Autodesk Inventor part; units mm, degrees
ref_plane "YZ Plane" through (0, 0, 0) normal (1, 0, 0) x (0, 1, 0)
ref_plane "XZ Plane" through (0, 0, 0) normal (0, 1, 0) x (-1, 0, 0)
ref_plane "XY Plane" through (0, 0, 0) normal (0, 0, 1) x (1, 0, 0)
sketch "Sketch1" plane through (0, 0, 0) normal (0, 1, 0) x (-1, 0, 0)
  line L0 (0, 0) -> (130, 0)
  line L1 (130, 0) -> (130, -100)
  line L2 (130, -100) -> (0, -100)
  line L3 (0, -100) -> (0, 0)
  dimension "d0" = 130
  dimension "d1" = 100
extrude "Extrusion1" add sketch "Sketch1" along normal blind 8
sketch "Sketch3" plane through (0, 8, 0) normal (0, 1, 0) x (1, 0, 0)
  line L0 (-120, 5) -> (-110, 5)
  line L1 (-110, 5) -> (-110, 15)
  line L2 (-110, 15) -> (-120, 15)
  line L3 (-120, 15) -> (-120, 5)
  line L4 (-130, 100) -> (-130, 0)
  line L5 (-130, 0) -> (0, 0)
  line L6 (-105, 0) -> (-105, 100)
  line L7 (0, 100) -> (-130, 100)
  line L8 (-130, 20) -> (-105, 20)
  line L9 (-120, 35) -> (-110, 35)
  line L10 (-110, 35) -> (-110, 25)
  line L11 (-110, 25) -> (-120, 25)
  line L12 (-120, 25) -> (-120, 35)
  line L13 (-130, 40) -> (-105, 40)
  line L14 (-120, 75) -> (-110, 75)
  line L15 (-110, 75) -> (-110, 65)
  line L16 (-110, 65) -> (-120, 65)
  line L17 (-120, 65) -> (-120, 75)
  line L18 (-120, 45) -> (-110, 45)
  line L19 (-110, 45) -> (-110, 55)
  line L20 (-110, 55) -> (-120, 55)
  line L21 (-120, 55) -> (-120, 45)
  line L22 (-130, 80) -> (-105, 80)
  line L23 (-120, 155) -> (-110, 155)
  line L24 (-110, 155) -> (-110, 145)
  line L25 (-110, 145) -> (-120, 145)
  line L26 (-120, 145) -> (-120, 155)
  line L27 (-130, 100) -> (0, 100)
  line L28 (-120, 125) -> (-110, 125)
  line L29 (-110, 125) -> (-110, 135)
  line L30 (-110, 135) -> (-120, 135)
  line L31 (-120, 135) -> (-120, 125)
  line L32 (-110, 95) -> (-120, 95)
  line L33 (-120, 95) -> (-120, 85)
  line L34 (-110, 105) -> (-120, 105)
  line L35 (-120, 85) -> (-110, 85)
  line L36 (-110, 85) -> (-110, 95)
  line L37 (-120, 105) -> (-120, 115)
  line L38 (-120, 115) -> (-110, 115)
  line L39 (-110, 115) -> (-110, 105)
  line L40 (-90, 5) -> (-100, 5)
  line L41 (-100, 5) -> (-100, 15)
  line L42 (-100, 15) -> (-90, 15)
  line L43 (-90, 15) -> (-90, 5)
  line L44 (-90, 35) -> (-100, 35)
  line L45 (-100, 35) -> (-100, 25)
  line L46 (-100, 25) -> (-90, 25)
  line L47 (-90, 25) -> (-90, 35)
  line L48 (-100, 65) -> (-90, 65)
  line L49 (-90, 65) -> (-90, 75)
  line L50 (-100, 55) -> (-90, 55)
  line L51 (-90, 75) -> (-100, 75)
  line L52 (-100, 75) -> (-100, 65)
  line L53 (-90, 55) -> (-90, 45)
  line L54 (-90, 45) -> (-100, 45)
  line L55 (-100, 45) -> (-100, 55)
  line L56 (-100, 105) -> (-90, 105)
  line L57 (-90, 105) -> (-90, 115)
  line L58 (-100, 115) -> (-100, 105)
  line L59 (-90, 115) -> (-100, 115)
  line L60 (-90, 125) -> (-100, 125)
  line L61 (-100, 125) -> (-100, 135)
  line L62 (-100, 135) -> (-90, 135)
  line L63 (-90, 135) -> (-90, 125)
  line L64 (-90, 155) -> (-100, 155)
  line L65 (-100, 155) -> (-100, 145)
  line L66 (-100, 145) -> (-90, 145)
  line L67 (-90, 145) -> (-90, 155)
  line L68 (-90, 95) -> (-90, 85)
  line L69 (-90, 85) -> (-100, 85)
  line L70 (-100, 85) -> (-100, 95)
  line L71 (-100, 95) -> (-90, 95)
  line L72 (-85, 0) -> (-85, 100)
  line L73 (-50, 5) -> (-60, 5)
  line L74 (-60, 5) -> (-60, 15)
  line L75 (-60, 15) -> (-50, 15)
  line L76 (-50, 15) -> (-50, 5)
  line L77 (-50, 35) -> (-60, 35)
  line L78 (-60, 35) -> (-60, 25)
  line L79 (-60, 25) -> (-50, 25)
  line L80 (-50, 25) -> (-50, 35)
  line L81 (-60, 65) -> (-50, 65)
  line L82 (-50, 65) -> (-50, 75)
  line L83 (-60, 55) -> (-50, 55)
  line L84 (-50, 75) -> (-60, 75)
  line L85 (-60, 75) -> (-60, 65)
  line L86 (-50, 55) -> (-50, 45)
  line L87 (-50, 45) -> (-60, 45)
  line L88 (-60, 45) -> (-60, 55)
  line L89 (-60, 105) -> (-50, 105)
  line L90 (-50, 105) -> (-50, 115)
  line L91 (-60, 115) -> (-60, 105)
  line L92 (-50, 115) -> (-60, 115)
  line L93 (-50, 125) -> (-60, 125)
  line L94 (-60, 125) -> (-60, 135)
  line L95 (-60, 135) -> (-50, 135)
  line L96 (-50, 135) -> (-50, 125)
  line L97 (-50, 155) -> (-60, 155)
  line L98 (-60, 155) -> (-60, 145)
  line L99 (-60, 145) -> (-50, 145)
  line L100 (-50, 145) -> (-50, 155)
  line L101 (-50, 95) -> (-50, 85)
  line L102 (-50, 85) -> (-60, 85)
  line L103 (-60, 85) -> (-60, 95)
  line L104 (-60, 95) -> (-50, 95)
  line L105 (-80, 125) -> (-70, 125)
  line L106 (-70, 125) -> (-70, 135)
  line L107 (-80, 135) -> (-80, 125)
  line L108 (-70, 135) -> (-80, 135)
  line L109 (-70, 145) -> (-80, 145)
  line L110 (-80, 155) -> (-70, 155)
  line L111 (-80, 145) -> (-80, 155)
  line L112 (-70, 155) -> (-70, 145)
  line L113 (-70, 15) -> (-80, 15)
  line L114 (-80, 15) -> (-80, 5)
  line L115 (-80, 5) -> (-70, 5)
  line L116 (-70, 5) -> (-70, 15)
  line L117 (-80, 45) -> (-70, 45)
  line L118 (-80, 35) -> (-70, 35)
  line L119 (-70, 25) -> (-80, 25)
  line L120 (-80, 25) -> (-80, 35)
  line L121 (-70, 35) -> (-70, 25)
  line L122 (-70, 45) -> (-70, 55)
  line L123 (-80, 55) -> (-80, 45)
  line L124 (-70, 65) -> (-80, 65)
  line L125 (-70, 75) -> (-70, 65)
  line L126 (-80, 65) -> (-80, 75)
  line L127 (-80, 75) -> (-70, 75)
  line L128 (-70, 55) -> (-80, 55)
  line L129 (-80, 85) -> (-70, 85)
  line L130 (-70, 85) -> (-70, 95)
  line L131 (-80, 95) -> (-80, 85)
  line L132 (-70, 95) -> (-80, 95)
  line L133 (-70, 105) -> (-80, 105)
  line L134 (-80, 115) -> (-70, 115)
  line L135 (-80, 105) -> (-80, 115)
  line L136 (-70, 115) -> (-70, 105)
  line L137 (-45, 0) -> (-45, 100)
  line L138 (-10, 125) -> (-20, 125)
  line L139 (-20, 125) -> (-20, 135)
  line L140 (-10, 135) -> (-10, 125)
  line L141 (-20, 135) -> (-10, 135)
  line L142 (-20, 145) -> (-10, 145)
  line L143 (-20, 155) -> (-20, 145)
  line L144 (-10, 155) -> (-20, 155)
  line L145 (-10, 145) -> (-10, 155)
  line L146 (-40, 5) -> (-30, 5)
  line L147 (-30, 5) -> (-30, 15)
  line L148 (-30, 15) -> (-40, 15)
  line L149 (-40, 15) -> (-40, 5)
  line L150 (-40, 65) -> (-40, 75)
  line L151 (-40, 35) -> (-30, 35)
  line L152 (-30, 35) -> (-30, 25)
  line L153 (-30, 25) -> (-40, 25)
  line L154 (-40, 25) -> (-40, 35)
  line L155 (-30, 65) -> (-40, 65)
  line L156 (-40, 75) -> (-30, 75)
  line L157 (-30, 75) -> (-30, 65)
  line L158 (-30, 55) -> (-40, 55)
  line L159 (-40, 55) -> (-40, 45)
  line L160 (-40, 45) -> (-30, 45)
  line L161 (-30, 45) -> (-30, 55)
  line L162 (-30, 125) -> (-30, 135)
  line L163 (-30, 155) -> (-30, 145)
  line L164 (-40, 125) -> (-30, 125)
  line L165 (-40, 135) -> (-40, 125)
  line L166 (-30, 135) -> (-40, 135)
  line L167 (-30, 145) -> (-40, 145)
  line L168 (-40, 145) -> (-40, 155)
  line L169 (-40, 155) -> (-30, 155)
  line L170 (-30, 105) -> (-40, 105)
  line L171 (-40, 105) -> (-40, 115)
  line L172 (-30, 115) -> (-30, 105)
  line L173 (-40, 115) -> (-30, 115)
  line L174 (-40, 95) -> (-40, 85)
  line L175 (-40, 85) -> (-30, 85)
  line L176 (-30, 85) -> (-30, 95)
  line L177 (-30, 95) -> (-40, 95)
  line L178 (-10, 115) -> (-20, 115)
  line L179 (-20, 115) -> (-20, 105)
  line L180 (-10, 105) -> (-10, 115)
  line L181 (-20, 105) -> (-10, 105)
  line L182 (-20, 95) -> (-10, 95)
  line L183 (-20, 85) -> (-20, 95)
  line L184 (-10, 85) -> (-20, 85)
  line L185 (-10, 95) -> (-10, 85)
  line L186 (-10, 75) -> (-20, 75)
  line L187 (-10, 65) -> (-10, 75)
  line L188 (-20, 65) -> (-10, 65)
  line L189 (-20, 75) -> (-20, 65)
  line L190 (-20, 15) -> (-10, 15)
  line L191 (-10, 15) -> (-10, 5)
  line L192 (-20, 5) -> (-20, 15)
  line L193 (-10, 5) -> (-20, 5)
  line L194 (-10, 45) -> (-20, 45)
  line L195 (-10, 35) -> (-20, 35)
  line L196 (-10, 25) -> (-10, 35)
  line L197 (-20, 25) -> (-10, 25)
  line L198 (-20, 55) -> (-10, 55)
  line L199 (-20, 45) -> (-20, 55)
  line L200 (-20, 35) -> (-20, 25)
  line L201 (-10, 55) -> (-10, 45)
  point P0 (-65, 20)
  point P1 (-65, 40)
  point P2 (-65, 80)
  point P3 (-25, 20)
  point P4 (-25, 40)
  point P5 (-25, 80)
  dimension "d21" = 10
  dimension "d22" = 10
  dimension "d23" = 10
  dimension "d24" = 5
  dimension "d25" = 5
  dimension "d26" = 5
  dimension "d27" = 5
  dimension "d28" = 5
  dimension "d29" = 5
  dimension "d30" = 5
  dimension "d40" = 5
sketch "Sketch4" plane through (0, 8, 0) normal (0, 1, 0) x (1, 0, 0)
  circle A0 centre (-120, 10) radius 3.5
  line L0 (-130, 0) -> (0, 0)
  line L1 (-130, 100) -> (-130, 0)
  line L2 (-65, 0) -> (-65, 170)
  line L3 (-130, 100) -> (-130, 0)
  line L4 (-130, 50) -> (0, 50)
  circle A1 centre (-10, 10) radius 3.5
  circle A2 centre (-120, 90) radius 3.5
  line L5 (-130, 100) -> (0, 100)
  circle A3 centre (-10, 90) radius 3.5
  point P0 (0, 100)
  dimension "d35" = 7
  dimension "d36" = 10
  dimension "d37" = 10
extrude "Extrusion5" cut sketch "Sketch4" against normal blind 20 contours A0 | A1 | A2 | A3
extrude "Extrusion6" cut sketch "Sketch3" against normal blind 20 contours L9 L10 L11 L12 | L14 L15 L16 L17 | L21 L20 L19 L18 | L47 L46 L45 L44 | L52 L51 L49 L48 | L50 L53 L54 L55 | L80 L79 L78 L77 | L85 L84 L82 L81 | L83 L86 L87 L88 | L123 L128 L122 L117 | L118 L121 L119 L120 | L124 L126 L127 L125 | L150 L156 L157 L155 | L151 L152 L153 L154 | L161 L160 L159 L158 | L187 L188 L189 L186 | L194 L199 L198 L201 | L196 L197 L200 L195
properties part number "floor_plan"
Model file for the job. Use its own axes, mm. Give positions to 0.01 mm unless a question says otherwise; leave off trailing zeros. Loops run counter-clockwise (first coordinate to the right, second up) from the corner with the lowest first, then second, coordinate; pieces in that order, holes last. Notation, with made-up numbers: (50, -34) -> (59, -34) arc R23 cw to (59, -12) -> close; hole circle Ø9 at (15.25, 6). An arc over 180 degrees is marked (long way). Use CSV: the item, a comma, the result in double quotes. Start each with the question number.
1) Slice it at B-B on x = -32. Give the cut face in (y, z), plus the area to 3 significant figures.
2) Slice it at D-D on x = -121.5. Give the cut face in (y, z).
3) Slice it at A-A on z = -10. Give the cut face in (x, y).
4) Mould opens along X. For faces 1 (the flat face through (-70, 4, -70)), 2 (the flat face through (-64, 4, 0)) say: released by +X, released by -X, zero draft, split by the parting line, or undercut.
5) Wall check: line 1 (Z direction, x = -92, y = 5.5); line 2 (X direction, y = 5.25, z = -10); line 3 (Z direction, x = -122.5, y = 4.25). Give the ranges that are in metal, low to high.
6) Slice it at C-C on z = -33.5. Give the cut face in (x, y).
Computed values:
1,outline,"(0, -100) -> (8, -100) -> (8, -75) -> (0, -75) -> close; (0, -65) -> (8, -65) -> (8, -55) -> (0, -55) -> close; (0, -45) -> (8, -45) -> (8, -35) -> (0, -35) -> close; (0, -25) -> (8, -25) -> (8, 0) -> (0, 0) -> close"
1,area,"560 mm^2"
2,outline,"(0, -100) -> (8, -100) -> (8, -93.16) -> (0, -93.16) -> close; (0, -86.84) -> (8, -86.84) -> (8, -13.16) -> (0, -13.16) -> close; (0, -6.84) -> (8, -6.84) -> (8, 0) -> (0, 0) -> close"
3,outline,"(-130, 0) -> (-123.5, 0) -> (-123.5, 8) -> (-130, 8) -> close; (-116.5, 0) -> (-13.5, 0) -> (-13.5, 8) -> (-116.5, 8) -> close; (-6.5, 0) -> (0, 0) -> (0, 8) -> (-6.5, 8) -> close"
4,face 1,"undercut"
4,face 2,"zero draft"
5,line 1,"z = -100 to -75, -65 to -55, -45 to -35, -25 to 0"
5,line 2,"x = -130 to -123.5, -116.5 to -13.5, -6.5 to 0"
5,line 3,"z = -100 to -92.45, -87.55 to -12.45, -7.55 to 0"
6,outline,"(-130, 0) -> (-120, 0) -> (-120, 8) -> (-130, 8) -> close; (-110, 0) -> (-100, 0) -> (-100, 8) -> (-110, 8) -> close; (-90, 0) -> (-80, 0) -> (-80, 8) -> (-90, 8) -> close; (-70, 0) -> (-60, 0) -> (-60, 8) -> (-70, 8) -> close; (-50, 0) -> (-40, 0) -> (-40, 8) -> (-50, 8) -> close; (-30, 0) -> (-20, 0) -> (-20, 8) -> (-30, 8) -> close; (-10, 0) -> (0, 0) -> (0, 8) -> (-10, 8) -> close"
